from build123d import *

# Parameters (mm, degrees)
CROQUIS1_W              = 70
CROQUIS1_H              = 30
SALIENTE_EXTRUIR1_DEPTH = 22
VACIADO1_T              = -2
CORTAR_EXTRUIR1_DEPTH   = 22
CORTAR_EXTRUIR3_DEPTH   = 22


with BuildPart() as part:
    # Croquis1 → Saliente-Extruir1 (new body)
    with BuildSketch(Plane(origin=(0, 0, 0), x_dir=(1, 0, 0), z_dir=(0, 1, 0))):
        with Locations((35, 15)):
            Rectangle(CROQUIS1_W, CROQUIS1_H)
    extrude(amount=SALIENTE_EXTRUIR1_DEPTH)

    # Vaciado1
    vaciado1_openings = [part.faces().sort_by_distance(p)[0] for p in [
        (35, 22, -15),
    ]]
    offset(amount=VACIADO1_T, openings=vaciado1_openings, kind=Kind.INTERSECTION)

    # Croquis2 → Cortar-Extruir1 (cut)
    with BuildSketch(Plane(origin=(0, 2, 0), x_dir=(1, 0, 0), z_dir=(0, 1, 0))):
        with BuildLine():
            Line((60, 17), (50, 17))
            ThreePointArc((50, 17), (48, 15), (50, 13))
            Line((50, 13), (60, 13))
            ThreePointArc((60, 13), (62, 15), (60, 17))
        make_face()
        with BuildLine():
            Line((10, 17), (20, 17))
            ThreePointArc((20, 17), (22, 15), (20, 13))
            Line((20, 13), (10, 13))
            ThreePointArc((10, 13), (8, 15), (10, 17))
        make_face()
    extrude(amount=-CORTAR_EXTRUIR1_DEPTH, mode=Mode.SUBTRACT)

    # Croquis3 → Cortar-Extruir3 (cut)
    with BuildSketch(Plane(origin=(0, 22, 0), x_dir=(1, 0, 0), z_dir=(0, 1, 0))):
        Polygon((2.056887166, 0), (0, 2.056887166), (0, 0), align=None)
        Polygon((70, 0), (70, 2.056887166), (67.943112834, 0), align=None)
        Polygon((70, 30), (67.943112834, 30), (70, 27.943112834), align=None)
        Polygon((0, 30), (2.056887166, 30), (0, 27.943112834), align=None)
    extrude(amount=-CORTAR_EXTRUIR3_DEPTH, mode=Mode.SUBTRACT)


solid = part.part
Here's how the part is built. I have some questions about the finished solid (model axes, mm). A direction names the side the tool comes from. Coordinates: 2 decimals unless noted, no trailing zeros. Order: outer loops, then holes, each group sorted by start corner. A loop starts at its lowest first (then second) coordinate and runs counter-clockwise, first axis right, second up. Notation, with made-up numbers: M -9.75,-6.5 L 41.25,-6.5 A33 cw 41.25,24.5 Z; hole C 49.25,19.25 d7. An arc over 180 degrees is marked long. Answer as CSV lines item,"result". Start each with the question number.
1. I want a section at B-B, the plane y = 16.5. Write out the boundary of the cut face in (x, z), and give its area (3 significant figures).
2. I want a section at A-A, the plane z = -15. Write out the boundary of the cut face in (x, y).
3. I need wall thicknesses on line 1 (X direction, y = 19.5, z = -20.75); line 2 (Z direction, x = 61.5, y = 2.5); line 3 (Y direction, x = 34, z = -3.5). Which ranges of each line are inside material? Lowest first, please. Write a range as [from, to].
4. We'd pull the mould along Z, two halves only. Please class faces 4 (the flat face through (35, 11, 0)), 5 (the flat face through (15, 1, -17)), 6 (the flat face through (1.043, 11.154, -28.986)), 7 (the flat face through (55, 1, -13)): released by +Z, released by -Z, zero draft, split by the parting line, or undercut.
5. On a 3-axis mill with a long thin cutter (end or side, diameter ignored), from which of +Z, -Z, +X, -X, +Y, -Y can I reach the whole of each face in a straight line? I mean faces 1 (the flat face through (35, 2, -15)), 2 (the cylindrical face through (22, 1, -15)), 3 (the flat face through (68.957, 11.154, -28.986)). Say none if no direction works.
6. I want a section at C-C, the plane x = 15. Write out the boundary of the cut face in (y, z).
7. I want a section at D-D, the plane x = 42.5. Write out the boundary of the cut face in (y, z).
8. For pin 1 (8 mm diameter, centred on x = 40, z = -11, fed in from +Y); pin 2 (1 mm diameter, centred on x = 13, z = -14.5, fed in from +Y), each with a flat end and sliding along its axis, tell me the tip position at first contact or that it passes through.
Recorded:
1,outline,"M 0,-27.94 L 2.06,-30 L 67.94,-30 L 70,-27.94 L 70,-2.06 L 67.94,0 L 2.06,0 L 0,-2.06 Z; hole M 2,-28 L 68,-28 L 68,-2 L 2,-2 Z"
1,area,"376 mm2"
2,outline,"M 0,0 L 8,0 L 8,2 L 2,2 L 2,22 L 0,22 Z; M 22,0 L 48,0 L 48,2 L 22,2 Z; M 62,0 L 70,0 L 70,22 L 68,22 L 68,2 L 62,2 Z"
3,line 1,"x = [0, 2], [68, 70]"
3,line 2,"z = [-30, -28], [-2, 0]"
3,line 3,"y = [0, 2]"
4,face 4,"released by +Z"
4,face 5,"undercut"
4,face 6,"released by -Z"
4,face 7,"undercut"
5,face 1,"+Y"
5,face 2,"+Y, -Y"
5,face 3,"-Z, +X, +Y, -Y"
6,outline,"M 0,-30 L 22,-30 L 22,-28 L 2,-28 L 2,-17 L 0,-17 Z; M 0,-13 L 2,-13 L 2,-2 L 22,-2 L 22,0 L 0,0 Z"
7,outline,"M 0,-30 L 22,-30 L 22,-28 L 2,-28 L 2,-2 L 22,-2 L 22,0 L 0,0 Z"
8,pin 1,"stops at y = 2"
8,pin 2,"passes through"
